Geometry: final body of the model. Coordinates: model frame, mm. Face numbers are marked on the shaded views. A direction names the side the tool comes from. Round coordinates to 2 decimals unless told otherwise and drop trailing zeros. Order: outer loops, then holes, each group sorted by start corner. A loop starts at its lowest first (then second) coordinate and runs counter-clockwise, first axis right, second up. Notation, with made-up numbers: M 26.25,67.25 L 84.25,67.25 A16 cw 84.25,95.25 Z; hole C 27,41 d4. An arc over 180 degrees is marked long. Return JSON: item names as keys, results as strings. Group by question number.
Q1. Cut plane A-A on x = 4. Output: boundary loops of the cut face in (y, z), and give its area (3 significant figures).
Q2. Ray query, probe 1 along X at (y, z) = (0, -1.75); probe 2 along Y at (x, z) = (16, -1.5); probe 3 along X at (y, z) = (0.5, 1.5). Return the intervals inside material, ascending.
Q3. Contact query for flat-ended pins moving along their axis: pin 1 (4 mm diameter, centred on x = 28.5, z = 0, fed in from +Y); pin 2 (1.5 mm diameter, centred on y = -2, z = 0, fed in from -X); pin 3 (3 mm diameter, centred on x = 21, y = 2.5, fed in from -Z). Output: stop coordinate, or through.
Q4. Access query for the marked faces 1 and 2. Directions: +Z, -Z, +X, -X, +Y, -Y. A direction counts if a zero-diameter tool reaches every point of the face in a straight line with its end or side. Return the directions, or none.
```python
from build123d import *


with BuildPart() as f1:
    # F0 (on Front) → F1 (revolve)
    with BuildSketch(Plane.XZ):
        with BuildLine():
            Line((41, 2.5), (0, 2.5))
            Line((0, 2.5), (0, 4))
            ThreePointArc((0, 4), (-2.828427, 2.828427), (-4, 0))
            Line((-4, 0), (46, 0))
            Line((46, 0), (46, 2))
            Line((46, 2), (45, 2))
            Line((45, 2), (45, 1.5))
            Line((45, 1.5), (44, 1.5))
            Line((44, 1.5), (44, 2))
            Line((44, 2), (41, 2))
            Line((41, 2), (41, 2.5))
        make_face()
    revolve(axis=Axis((18.891413, 0, 0), (1, 0, 0)))


solid = f1.part
```
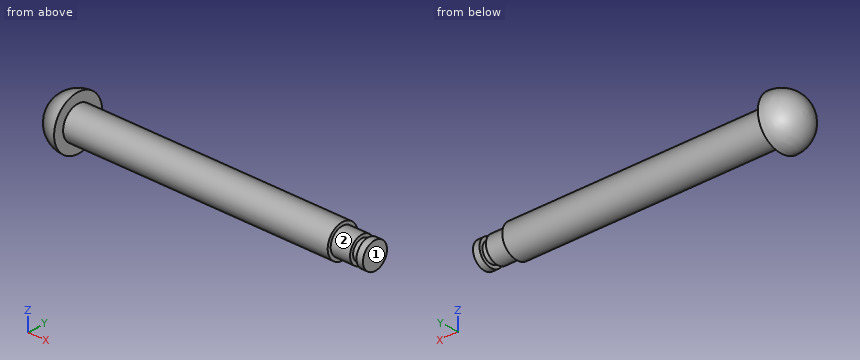
Result sheet:
{
 "1": {"outline": "C 0,0 d5", "area": "19.6 mm²"},
 "2": {"probe 1": "x = -3.6 to 44, 45 to 46", "probe 2": "y = -2 to 2", "probe 3": "x = -3.67 to 44, 45 to 46"},
 "3": {"pin 1": "stops at y = 2.5", "pin 2": "stops at x = -3.8", "pin 3": "stops at z = -2.29"},
 "4": {"face 1": "+Z, -Z, +X, +Y, -Y", "face 2": "+X"}
}
